Design review of the part built by this model. Coordinates are the model's own, in mm. Face numbers are marked on the shaded views. A direction names the side the tool comes from. Give positions to 0.01 mm unless a question says otherwise; leave off trailing zeros. Loops run counter-clockwise (first coordinate to the right, second up) from the corner with the lowest first, then second, coordinate; pieces in that order, holes last. Notation, with made-up numbers: (-4.75, -23.75) -> (6.25, -23.75) arc R19 cw to (6.25, 4.25) -> close; hole circle Ø11 at (89.5, -32). An arc over 180 degrees is marked (long way). Use CSV: the item, a comma, the result in double quotes. Start each with the question number.
Item 1: The part is to be moulded in two halves that separate along Y. For the marked faces 1, 2, 3 and 4, say which applies: +Y half, -Y half, draft (parallel to the pull), parting line (faces both ways), or undercut.
Item 2: We need section C-C (z = 8.25). State the section outline as (x, y) points.
Item 3: For the marked faces 5, 6 and 7, list the 3-axis set-ups (+Z, -Z, +X, -X, +Y, -Y) from which the entire face can be reached by the end or side of a thin tool; tool diameter is ignored.
Item 4: We need section A-A (z = 4). State the section outline as (x, y) points.
Item 5: We need section B-B (x = 17). State the section outline as (y, z) points, plus the area to 3 significant figures.
Item 6: Wall thickness on line 1 along X through (y, z) = (7, 5.5); line 2 along Z through (x, y) = (14.25, 17.25): over which ranges is each line inside the solid? List them lowest first. Write a range as from..to.
from build123d import *

# Parameters (mm, degrees)
SKETCH_W        = 20
SKETCH_H        = 20
PAD_DEPTH       = 15
SKETCH001_W     = 16
SKETCH001_H     = 16
POCKET_DEPTH    = 12
POCKET001_DEPTH = 20


with BuildPart() as part:
    # Sketch → Pad (new body)
    with BuildSketch(Plane.XY):
        with Locations((10, 10)):
            Rectangle(SKETCH_W, SKETCH_H)
    extrude(amount=PAD_DEPTH)

    # Sketch001 (on Face6 of Pad) → Pocket (cut)
    with BuildSketch(Plane.XY.offset(15)):
        with Locations((10, 10)):
            Rectangle(SKETCH001_W, SKETCH001_H)
    extrude(amount=-POCKET_DEPTH, mode=Mode.SUBTRACT)

    # Sketch002 (on Face3 of Pocket) → Pocket001 (cut)
    with BuildSketch(Plane.YZ.offset(20)):
        with BuildLine():
            ThreePointArc((12.5, 15.5), (10, 18), (7.5, 15.5))
            Line((7.5, 15.5), (7.5, 5.5))
            ThreePointArc((7.5, 5.5), (10, 3), (12.5, 5.5))
            Line((12.5, 5.5), (12.5, 15.5))
        make_face()
    extrude(amount=-POCKET001_DEPTH, mode=Mode.SUBTRACT)


solid = part.part
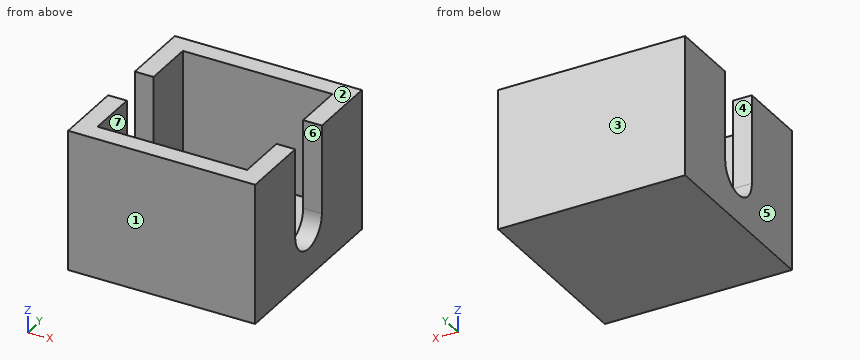
Results found:
1,face 1,"-Y half"
1,face 2,"draft"
1,face 3,"+Y half"
1,face 4,"undercut"
2,outline,"(0, 0) -> (20, 0) -> (20, 7.5) -> (18, 7.5) -> (18, 2) -> (2, 2) -> (2, 7.5) -> (0, 7.5) -> close; (0, 12.5) -> (2, 12.5) -> (2, 18) -> (18, 18) -> (18, 12.5) -> (20, 12.5) -> (20, 20) -> (0, 20) -> close"
3,face 5,"+Z, -Z, -X, +Y, -Y"
3,face 6,"+Z, +X, -X"
3,face 7,"+Z"
4,outline,"(0, 0) -> (20, 0) -> (20, 8) -> (18, 8) -> (18, 2) -> (2, 2) -> (2, 8) -> (0, 8) -> close; (0, 12) -> (2, 12) -> (2, 18) -> (18, 18) -> (18, 12) -> (20, 12) -> (20, 20) -> (0, 20) -> close"
5,outline,"(0, 0) -> (20, 0) -> (20, 15) -> (18, 15) -> (18, 3) -> (2, 3) -> (2, 15) -> (0, 15) -> close"
5,area,"108 mm²"
6,line 1,"0..2, 18..20"
6,line 2,"0..3"
